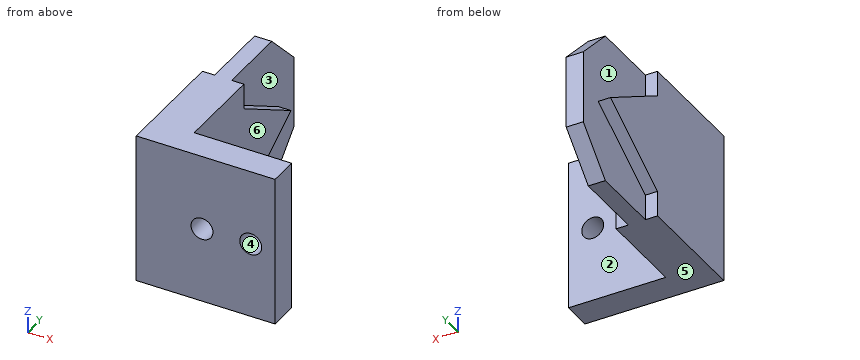
Autodesk Inventor part; units mm, degrees
ref_plane "YZ Plane" through (0, 0, 0) normal (1, 0, 0) x (0, 1, 0)
ref_plane "XZ Plane" through (0, 0, 0) normal (0, 1, 0) x (-1, 0, 0)
ref_plane "XY Plane" through (0, 0, 0) normal (0, 0, 1) x (1, 0, 0)
sketch "Sketch1" plane through (0, 0, 0) normal (1, 0, 0) x (0, 1, 0)
  line L0 (22.5, 15.5) -> (0, 15.5)
  line L1 (0, 15.5) -> (0, -15.5)
  line L2 (0, -15.5) -> (22.5, -15.5)
  line L3 (22.5, -15.5) -> (22.5, 15.5)
  line L4 (0, -21.7) -> (0, 21.7)
  point P0 (0, 0)
  point P1 (22.5, 0)
  dimension "d0" = 31
  dimension "d1" = 22.5
extrude "Extrusion1" add sketch "Sketch1" along normal mid plane 3.5
sketch "Sketch2" plane through (1.75, 0, 0) normal (1, 0, 0) x (0, 0, -1)
  line L0 (-10.2455, 0) -> (0, 17.076)
  line L1 (0, 17.076) -> (10.2455, 0)
  line L2 (-15.5, 0) -> (15.5, 0)
  point P0 (0, 0)
  dimension "d31" = 20.491
  dimension "d33" = 17.076
extrude "Extrusion4" add sketch "Sketch2" along normal blind 2.5
mirror "Mirror2" about plane through (0, 0, 0) normal (1, 0, 0) of "Extrusion4"
sketch "Sketch7" plane through (-1.75, 0, -15.5) normal (0, -1, 0) x (1, 0, 0)
  line L0 (0, 0) -> (3.5, 0)
  line L1 (3.5, 5.2545) -> (3.5, 0)
  line L2 (3.5, 5.2545) -> (6, 5.2545)
  line L3 (6, 25.7455) -> (6, 5.2545)
  line L4 (3.5, 25.7455) -> (6, 25.7455)
  line L5 (3.5, 31) -> (3.5, 25.7455)
  line L6 (0, 31) -> (3.5, 31)
  line L7 (0, 25.7455) -> (0, 31)
  line L8 (0, 25.7455) -> (-2.5, 25.7455)
  line L9 (-2.5, 25.7455) -> (-2.5, 5.2545)
  line L10 (0, 5.2545) -> (-2.5, 5.2545)
  line L11 (0, 0) -> (0, 5.2545)
  point P0 (1.75, 15.5)
extrude "Extrusion5" add sketch "Sketch7" along normal blind 24
sketch "Sketch8" plane through (4.25, 0, -10.2455) normal (0, 0, -1) x (-1, 0, 0)
  line L0 (2.5, 0) -> (0, 0)
  line L1 (0, 0) -> (0, -24)
  line L2 (2.5, -24) -> (0, -24)
  line L3 (2.5, 0) -> (2.5, -24)
  point P0 (4.25, 0)
extrude "Extrusion6" add sketch "Sketch8" along normal up to surface (5.2545 mm away)
mirror "Mirror3" about plane through (0, 0, 0) normal (0, 0, 1) of "Extrusion6"
mirror "Mirror4" about plane through (0, 0, 0) normal (1, 0, 0) of "Extrusion6", "Mirror3"
sketch "Sketch9" plane through (4.25, 0, 0) normal (1, 0, 0) x (0, 0, -1)
  line L0 (0, 17.076) -> (-10.2455, 0) construction
  line L1 (0, 17.076) -> (0, -24) construction
  line L2 (-15.5, -24) -> (15.5, -24) construction
  line L3 (-5.1228, 8.538) -> (5.1227, 8.538) construction
  line L4 (0, 17.076) -> (10.2455, 0) construction
  line L5 (-7.5227, 4.538) -> (7.5227, 4.538) construction
  line L6 (-13.5227, -5.462) -> (13.5227, -5.462) construction
  point P0 (0, 0)
  dimension "d40" = 4
  dimension "d50" = 10
chamfer "Chamfer1" distance 8 angle 45 2 edges at (0, 22.5, 15.5) (0, 22.5, -15.5)
sketch "Sketch10" plane through (-1.75, -24, -15.5) normal (0, -1, 0) x (1, 0, 0)
  line L0 (6, 31) -> (6, 0)
  line L1 (6, 0) -> (26, 0)
  line L2 (26, 0) -> (26, 31)
  line L3 (26, 31) -> (6, 31)
  line L4 (6, 31) -> (6, 0)
  circle A0 centre (21, 15.5) radius 2.25
  circle A1 centre (11, 15.5) radius 2.25
  line L5 (16, 0) -> (16, 31) construction
  point P0 (1.75, 15.5)
  dimension "d63" = 20
  dimension "d64" = 4.5
  dimension "d65" = 10
extrude "Extrusion7" add sketch "Sketch10" against normal blind 6
properties part number "Traingular Hopper Connector v.2"
CAD build for the part. Positions are in the model's coordinates, mm. Face numbers are marked on the shaded views. A direction names the side the tool comes from. Round coordinates to 2 decimals unless told otherwise and drop trailing zeros. Order: outer loops, then holes, each group sorted by start corner. A loop starts at its lowest first (then second) coordinate and runs counter-clockwise, first axis right, second up. Notation, with made-up numbers: (-23.75, -27.5) - (1.25, -27.5) arc R17 ccw to (1.25, -20.5) - close; hole circle Ø1 at (46, -1.5). An arc over 180 degrees is marked (long way). Return JSON: item names as keys, results as strings.
(1) Pin check, flat tips, straight feed: pin 1 Ø1 at (y, z) = (0, 7) entering from +X; pin 2 Ø2 at (x, z) = (2.5, 11.5) entering from +Y; pin 3 Ø1.2 at (x, z) = (-3.5, -13.5) entering from +Y. Stop position of each tip, or through.
Answer key:
{"pin 1": "stops at x = 4.25", "pin 2": "stops at y = 19.16", "pin 3": "stops at y = 0"}
(2) Cut at A-A (x = 19.25). Give the cut face in (y, z), then the cut area to 3 significant figures.
Answer key:
{"outline": "(-24, -15.5) - (-18, -15.5) - (-18, -2.25) - (-24, -2.25) - close; (-24, 2.25) - (-18, 2.25) - (-18, 15.5) - (-24, 15.5) - close", "area": "159 mm^2"}
(3) Cut at D-D (x = 12.25). Give the cut face in (y, z), then the cut area to 3 significant figures.
Answer key:
{"outline": "(-24, -15.5) - (-18, -15.5) - (-18, 15.5) - (-24, 15.5) - close", "area": "186 mm^2"}
(4) Cut at B-B (z = -12.5). Give the cut face in (x, y), then the cut area to 3 significant figures.
Answer key:
{"outline": "(-4.25, -24) - (24.25, -24) - (24.25, -18) - (4.25, -18) - (4.25, 0) - (1.75, 0) - (1.75, 17.5) - (-1.75, 17.5) - (-1.75, 0) - (-4.25, 0) - close", "area": "385 mm^2"}
(5) Wall check: probe 1 along Z at (x, y) = (9.25, -22.55); probe 2 along X at (y, z) = (18.5, 5); probe 3 along Y at (x, z) = (-2.25, 12). Give the ranges that are in metal, low to high. Write a range as from..to.
Answer key:
{"probe 1": "z = -15.5..-2.25, 2.25..15.5", "probe 2": "x = -1.75..1.75", "probe 3": "y = -24..0"}
(6) Cut at C-C (y = 4.5). Give the cut face in (x, z).
Answer key:
{"outline": "(-4.25, -7.55) - (-1.75, -7.55) - (-1.75, -15.5) - (1.75, -15.5) - (1.75, -7.55) - (4.25, -7.55) - (4.25, 7.55) - (1.75, 7.55) - (1.75, 15.5) - (-1.75, 15.5) - (-1.75, 7.55) - (-4.25, 7.55) - close"}
(7) Tool access for the marked faces 1, 2 and 3: list every direction of +Z, -Z, +X, -X, +Y, -Y with a clear straight run to the whole face (end or side of a thin tool).
Answer key:
{"face 1": "-X, +Y", "face 2": "+Z, -Z, +X, +Y", "face 3": "+X, +Y"}
(8) Pull direction Z, two halves, no side cores. Call the marked faces 4, 5 and 6: +Z half, -Z half, draft (parallel to the pull), parting line (faces both ways), or undercut.
Answer key:
{"face 4": "undercut", "face 5": "-Z half", "face 6": "draft"}
